```python
from build123d import *

# Parameters (mm, degrees)
SKETCH1_R          = 9
SKETCH1_R_2        = 5.25
BASE_EXTRUDE_DEPTH = 0.5
TYPEASLOT_DEPTH    = 13.737739203
TYPEAPATTERN_COUNT = 9


with BuildPart() as part:
    # Sketch1 → Base-Extrude (new body)
    with BuildSketch(Plane(origin=(0, 0, 0), x_dir=(0, 0, -1), z_dir=(1, 0, 0))):
        Circle(SKETCH1_R)
        Circle(SKETCH1_R_2, mode=Mode.SUBTRACT)
    extrude(amount=-BASE_EXTRUDE_DEPTH)

    # Sketch3 → TypeASlot (cut, through all)
    with BuildSketch(Plane(origin=(0, 0, 0), x_dir=(0, 0, -1), z_dir=(1, 0, 0))):
        with BuildLine():
            Line((0.732571764, 7.589401083), (1.35, 8.89817397))
            Line((1.35, 8.89817397), (1.35, 9.70817397))
            Line((1.35, 9.70817397), (-1.35, 9.70817397))
            Line((-1.35, 9.70817397), (-1.35, 8.89817397))
            Line((-1.35, 8.89817397), (-0.732571764, 7.589401083))
            ThreePointArc((-0.732571764, 7.589401083), (0, 7.125), (0.732571764, 7.589401083))
        make_face()
    typeaslot = extrude(amount=-TYPEASLOT_DEPTH, mode=Mode.SUBTRACT)

    # TypeAPattern: TypeASlot ×9 about axis
    typeapattern_axis = Axis((0, 0, 0), (1, 0, 0))
    for i in range(1, TYPEAPATTERN_COUNT):
        add(typeaslot.rotate(typeapattern_axis, i * 360 / TYPEAPATTERN_COUNT), mode=Mode.SUBTRACT)


solid = part.part
```
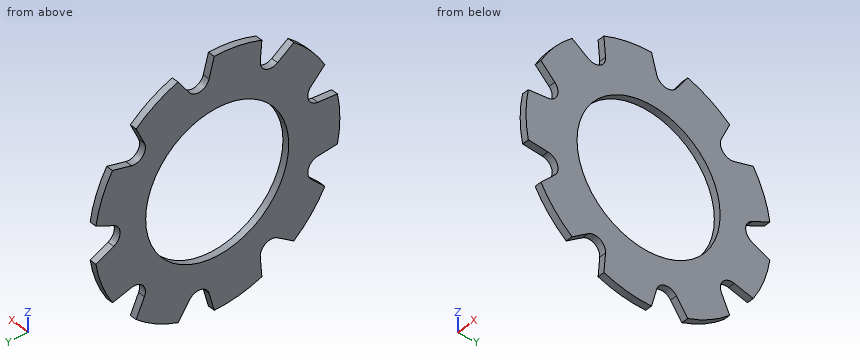
Could you check a few things on this model? Use its own coordinates, in mm. Round coordinates to 2 decimals unless told otherwise and drop trailing zeros. Loops run counter-clockwise (first coordinate to the right, second up) from the corner with the lowest first, then second, coordinate; pieces in that order, holes last. Notation, with made-up numbers: (16.5, 72) - (65.5, 72) arc R18 ccw to (65.5, 80) - close; hole circle Ø2 at (39, -21). An arc over 180 degrees is marked (long way). Answer as CSV lines item,"result".
1. I want a section at B-B on y = 0. List the corners of the cut face in (x, z) for me, then the cut area to 3 significant figures.
Filled in:
outline,"(-0.5, -9) - (0, -9) - (0, -5.25) - (-0.5, -5.25) - close; (-0.5, 5.25) - (0, 5.25) - (0, 9) - (-0.5, 9) - close"
area,"3.75 mm^2"
2. Please list where these lines run through material, in increasing order: line 1 along Z through (x, y) = (-0.15, 6); line 2 along Z through (x, y) = (-0.3, 4); line 3 along Y through (x, z) = (-0.05, 3.75). Write a range as [from, to].
Filled in:
line 1,"z = [-4.29, 4.29]"
line 2,"z = [-8.06, -3.4], [3.4, 8.06]"
line 3,"y = [-7.34, -3.67], [3.67, 8.18]"
3. For pin 1 Ø8 at (y, z) = (-4, -1) entering from -X; pin 2 Ø9.5 at (y, z) = (0, 0) entering from -X, each with a flat end and sliding along its axis, tell me the tip position at first contact or that it passes through.
Filled in:
pin 1,"stops at x = -0.5"
pin 2,"passes through"
4. I want a section at A-A on z = 0. List the corners of the cut face in (x, y) for me (3 decimals), then the cut area to 3 significant figures.
Filled in:
outline,"(-0.5, -9) - (0, -9) - (0, -5.25) - (-0.5, -5.25) - close; (-0.5, 5.25) - (0, 5.25) - (0, 7.125) - (-0.5, 7.125) - close"
area,"2.81 mm^2"
